```python
from build123d import *

# Parameters (mm, degrees)
SKETCH_1_W          = 35
SKETCH_1_H          = 35
EXTRUDE_1_DEPTH     = 5
EXTRUDE_2_DEPTH     = 7.3
EXTRUDE_START       = -7.3
EXTRUDE_3_DEPTH     = 7.3
SKETCH_4_W          = 35
SKETCH_4_H          = 45
EXTRUDE_4_DEPTH     = 5
SKETCH_6_R          = 6.1
CUT_EXTRUDE_1_DEPTH = 46.051329388
SKETCH_7_R          = 6.1
CUT_EXTRUDE_2_DEPTH = 46.051329388
SKETCH_8_R          = 1.6
CUT_EXTRUDE_3_DEPTH = 10


with BuildPart() as part:
    # 草图1 → 凸台-拉伸1 (new body)
    with BuildSketch(Plane.XY):
        Rectangle(SKETCH_1_W, SKETCH_1_H)
    extrude(amount=EXTRUDE_1_DEPTH)

    # 草图2 → 凸台-拉伸2 (add)
    with BuildSketch(Plane.ZY.offset(17.5)):
        with BuildLine():
            Line((5, 17.5), (-10, 17.5))
            Line((-10, 17.5), (-10, 17.496950369))
            ThreePointArc((-10, 17.496950369), (-27.496950369, 0), (-10, -17.496950369))
            Line((-10, -17.496950369), (-10, -17.5))
            Line((-10, -17.5), (5, -17.5))
            Line((5, -17.5), (5, 17.5))
        make_face()
    extrude(amount=-EXTRUDE_2_DEPTH)

    # 草图3 → 凸台-拉伸3 (add)
    with BuildSketch(Plane(origin=(17.5, 0, 0), x_dir=(0, 0, -1), z_dir=(1, 0, 0)).offset(EXTRUDE_START)):
        with BuildLine():
            Line((10, 17.5), (-5, 17.5))
            Line((-5, 17.5), (-5, -17.5))
            Line((-5, -17.5), (10, -17.5))
            Line((10, -17.5), (10, -17.496950369))
            ThreePointArc((10, -17.496950369), (27.496950369, 0), (10, 17.496950369))
            Line((10, 17.496950369), (10, 17.5))
        make_face()
    extrude(amount=EXTRUDE_3_DEPTH)

    # 草图4 → 凸台-拉伸4 (add)
    with BuildSketch(Plane.XY.offset(5)):
        Rectangle(SKETCH_4_W, SKETCH_4_H)
    extrude(amount=-EXTRUDE_4_DEPTH)

    # 草图6 → 切除-拉伸1 (cut, through all)
    with BuildSketch(Plane(origin=(-10.2, 0, 0), x_dir=(0, 0, -1), z_dir=(1, 0, 0))):
        with Locations((9.880544607, 0)):
            Circle(SKETCH_6_R)
    extrude(amount=-CUT_EXTRUDE_1_DEPTH, mode=Mode.SUBTRACT)

    # 草图7 → 切除-拉伸2 (cut, through all)
    with BuildSketch(Plane.ZY.offset(-10.2)):
        with Locations(Location((-9.880544607, 0, 0), (0, 0, 180))):
            Circle(SKETCH_7_R)
    extrude(amount=-CUT_EXTRUDE_2_DEPTH, mode=Mode.SUBTRACT)

    # 草图8 → 切除-拉伸3 (cut)
    with BuildSketch(Plane(origin=(0, 0, 0), x_dir=(-1, 0, 0), z_dir=(0, 0, -1))):
        with Locations((0, 20)):
            Circle(SKETCH_8_R)
        with Locations((0, -20)):
            Circle(SKETCH_8_R)
    extrude(amount=-CUT_EXTRUDE_3_DEPTH, mode=Mode.SUBTRACT)


solid = part.part
```
The model under review builds one solid part; all positions refer to its coordinate system, in mm. A direction names the side the tool comes from. Round coordinates to 2 decimals unless told otherwise and drop trailing zeros. Loops run counter-clockwise (first coordinate to the right, second up) from the corner with the lowest first, then second, coordinate; pieces in that order, holes last. Notation, with made-up numbers: (-33.5, 87.5) -> (-11.5, 87.5) arc R22 cw to (-11.5, 109.5) -> close; hole circle Ø11 at (38.5, 3). An arc over 180 degrees is marked (long way). Answer as a JSON object with one key per item and string values. Group by question number.
1) For pin 1 Ø10.5 at (x, y) = (2.5, -2.5) entering from -Z; pin 2 Ø3.5 at (x, z) = (-15.5, -6.5) entering from +Y; pin 3 Ø7.5 at (y, z) = (0, -9.88) entering from +X; pin 4 Ø1.5 at (x, y) = (12, -14.5) entering from -Z, all flat-tipped, find the tip position at first contact; note any pin that passes through.
2) For faces 4 (the face through (0, 22.5, 3)), 5 (the face through (14, 17.5, -5)), 6 (the face through (-13.799, 0.268, -3.786)), 7 (the face through (-10.2, 0, -17)), 8 (the face through (-14, -17.5, -5)), list the 3-axis set-ups (+Z, -Z, +X, -X, +Y, -Y) from which the entire face can be reached by the end or side of a thin tool; tool diameter is ignored.
3) We need section B-B on x = 0. Write out the cut boundary in (y, z), then the cut area to 3 significant figures.
4) For line 1 (Y direction, x = 0, z = 2); line 2 (X direction, y = 9, z = -14.5); line 3 (Z direction, x = -8, y = 18), list the stretches that pass through material, from the lowest coordinate up. Write a range as [from, to].
5) We need section D-D on y = 0. Write out the cut boundary in (x, z), then the cut area to 3 significant figures.
6) We need section A-A on y = -20. Write out the cut boundary in (x, z).
7) Mouldability with a two-part tool opening along X and no side actions: class faces 1 (the face through (13.799, -0.268, -3.786)), 2 (the face through (-17.5, 5, -4)), 3 (the face through (0, 0, 0)) as released by +X, released by -X, zero draft, split by the parting line, or undercut.
Result set:
{
 "1": {"pin 1": "z = 0", "pin 2": "y = 17.5", "pin 3": "through", "pin 4": "z = -20.82"},
 "2": {"face 4": "+Z, -Z, +X, -X, +Y", "face 5": "-Z, +X, -X, +Y", "face 6": "+X, -X", "face 7": "-Z, +Y, -Y", "face 8": "-Z, +X, -X, -Y"},
 "3": {"outline": "(-22.5, 0) -> (-21.6, 0) -> (-21.6, 5) -> (-22.5, 5) -> close; (-18.4, 0) -> (18.4, 0) -> (18.4, 5) -> (-18.4, 5) -> close; (21.6, 0) -> (22.5, 0) -> (22.5, 5) -> (21.6, 5) -> close", "area": "193 mm²"},
 "4": {"line 1": "[-22.5, -21.6], [-18.4, 18.4], [21.6, 22.5]", "line 2": "[-17.5, -10.2], [10.2, 17.5]", "line 3": "[0, 5]"},
 "5": {"outline": "(-17.5, -27.5) -> (-10.2, -27.5) -> (-10.2, -15.98) -> (-17.5, -15.98) -> close; (-17.5, -3.78) -> (-10.2, -3.78) -> (-10.2, 0) -> (10.2, 0) -> (10.2, -3.78) -> (17.5, -3.78) -> (17.5, 5) -> (-17.5, 5) -> close; (10.2, -27.5) -> (17.5, -27.5) -> (17.5, -15.98) -> (10.2, -15.98) -> close", "area": "398 mm²"},
 "6": {"outline": "(-17.5, 0) -> (-1.6, 0) -> (-1.6, 5) -> (-17.5, 5) -> close; (1.6, 0) -> (17.5, 0) -> (17.5, 5) -> (1.6, 5) -> close"},
 "7": {"face 1": "zero draft", "face 2": "released by -X", "face 3": "undercut"}
}
